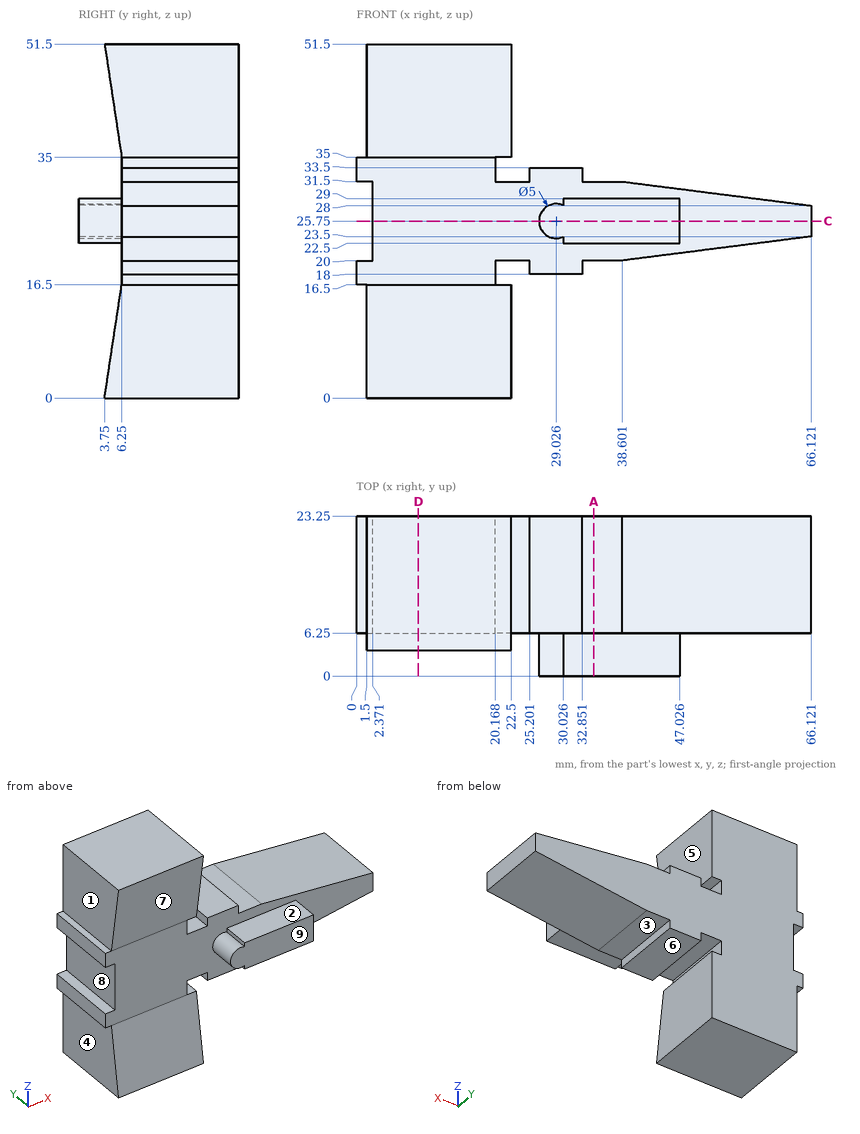
Could you check a few things on this drawing? It's one solid part, dimensions in mm from its lowest x, y, z. A direction names the side the tool comes from. Give positions to 0.01 mm unless a question says otherwise; leave off trailing zeros. Order: outer loops, then holes, each group sorted by start corner. A loop starts at its lowest first (then second) coordinate and runs counter-clockwise, first axis right, second up. Notation, with made-up numbers: (-2.75, 89) -> (17.25, 89) arc R12 ccw to (17.25, 103) -> close; hole circle Ø9 at (37, 66.25). An arc over 180 degrees is marked (long way). Answer in a Markdown table with one row per item. Add a question column.
Item 1: Imagine slicing it at A-A (x = 34.5). List the corners of the cut face in (y, z) for me, and give its area (3 significant figures).
Item 2: For the marked faces 1, 2, 3, 4 and 5, which set-ups out of +Z, -Z, +X, -X, +Y, -Y let a thin tool reach every point of the face, with its end or its side?
Item 3: We'd pull the mould along Z, two halves only. Please class the marked faces 6, 7, 8 and 9: pulls with the +Z half, pulls with the -Z half, needs draft (parallel to the pull), parting line crosses it, or undercut.
Item 4: Imagine slicing it at C-C (z = 25.75). List the corners of the cut face in (x, y) for me, and give its area (3 significant figures).
Item 5: I'm going to push flat-ended pins straight in: P1, Ø1.5, axis at y = 16, z = 18.5, coming from the +X side; P2, Ø8, axis at x = 34.5, y = 2.5, coming from the +Z side; P3, Ø6, axis at x = 29.5, y = 5.5, coming from the -Z side; P4, Ø2, axis at x = 49.5, z = 32.5, coming from the +Y side. Where does each tip first touch, or does it pass through?
Item 6: Please list where these lines run through material, in increasing order: probe 1 along X at (y, z) = (7.75, 35.5); probe 2 along Y at (x, z) = (13.5, 29); probe 3 along Z at (x, y) = (37, 19).
Item 7: Imagine slicing it at D-D (x = 9). List the corners of the cut face in (y, z) for me.
Result:
| question | item | result |
|---|---|---|
| 1 | outline | (0, 22.5) -> (6.25, 22.5) -> (6.25, 20) -> (23.25, 20) -> (23.25, 31.5) -> (6.25, 31.5) -> (6.25, 29) -> (0, 29) -> close |
| 1 | area | 236 mm2 |
| 2 | face 1 | +Z, -X, +Y, -Y |
| 2 | face 2 | +Z, +X, -X, -Y |
| 2 | face 3 | -Z, +X, +Y, -Y |
| 2 | face 4 | -Z, -X, +Y, -Y |
| 2 | face 5 | +Z, +X, +Y, -Y |
| 3 | face 6 | pulls with the -Z half |
| 3 | face 7 | undercut |
| 3 | face 8 | undercut |
| 3 | face 9 | needs draft |
| 4 | outline | (2.37, 6.25) -> (26.53, 6.25) -> (26.53, 0) -> (47.03, 0) -> (47.03, 6.25) -> (66.12, 6.25) -> (66.12, 23.25) -> (2.37, 23.25) -> close |
| 4 | area | 1,210 mm2 |
| 5 | P1 | x = 32.85 |
| 5 | P2 | z = 31.5 |
| 5 | P3 | z = 18 |
| 5 | P4 | through |
| 6 | probe 1 | 1.5 to 22.5 |
| 6 | probe 2 | 6.25 to 23.25 |
| 6 | probe 3 | 20 to 31.5 |
| 7 | outline | (3.75, 0) -> (23.25, 0) -> (23.25, 51.5) -> (3.75, 51.5) -> (6.25, 35) -> (6.25, 16.5) -> close |
